Print and shaded views of the part. All mm, measured from the part's lowest x, y and z. A direction names the side the tool comes from. Coordinates: 2 decimals unless noted, no trailing zeros. Loops run counter-clockwise (first coordinate to the right, second up) from the corner with the lowest first, then second, coordinate; pieces in that order, holes last. Notation, with made-up numbers: M -4.5,16 L 5.5,16 A18 ccw 5.5,45 Z; hole C -3,30 d10. An arc over 180 degrees is marked long. Answer as a JSON object with one key per item and string values. Group by question number.
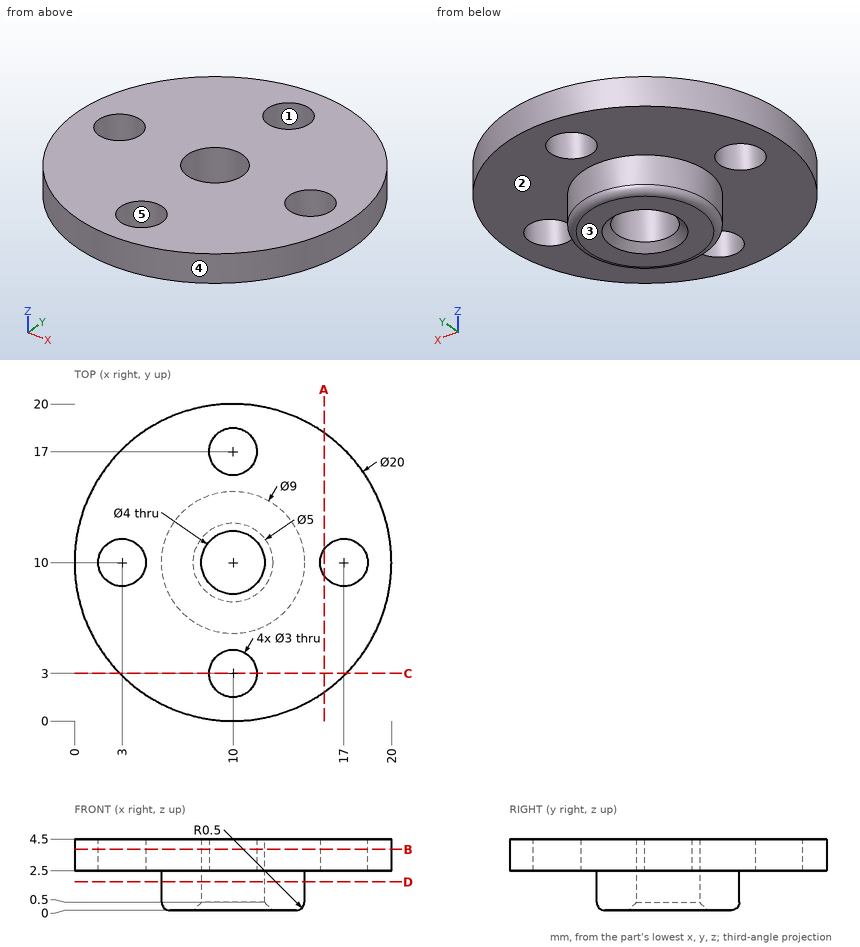
Item 1: Slice it at A-A, the plane x = 15.75. Write the cut outline in (y, z), then the cut area to 3 significant figures.
Item 2: Tool access for the marked faces 1 and 2: list every direction of +Z, -Z, +X, -X, +Y, -Y with a clear straight run to the whole face (end or side of a thin tool).
Item 3: Slice it at B-B, the plane z = 3.85. Write the cut outline in (x, y).
Item 4: Drill centre lines: L1, parallel to Z at x = 8.5, y = 15.25; L2, parallel to X at y = 2, z = 3.8; L3, parallel to Y at x = 10, z = 2.05. Where is each one in solid material? Low to high. Write a range as from..to.
Item 5: Slice it at D-D, the plane z = 1.8. Write the cut outline in (x, y).
Item 6: Pull direction Y, two halves, no side cores. Call the marked faces 3, 4 and 5: released by +Y, released by -Y, zero draft, split by the parting line, or undercut.
Item 7: Slice it at C-C, the plane y = 3. Write the cut outline in (x, z).
Item 8: Pin check, flat tips, straight feed: pin 1 (4 mm diameter, centred on x = 10, y = 17, fed in from -Z); pin 2 (1 mm diameter, centred on y = 7.5, z = 0.5, fed in from +X); pin 3 (2 mm diameter, centred on y = 6, z = 2.5, fed in from -X). Stop position of each tip, or through.
Computed:
{
 "1": {"outline": "M 1.82,2.5 L 9.17,2.5 L 9.17,4.5 L 1.82,4.5 Z; M 10.83,2.5 L 18.18,2.5 L 18.18,4.5 L 10.83,4.5 Z", "area": "29.4 mm2"},
 "2": {"face 1": "+Z, -Z", "face 2": "-Z"},
 "3": {"outline": "C 10,10 d20; hole C 3,10 d3; hole C 10,10 d4; hole C 10,3 d3; hole C 10,17 d3; hole C 17,10 d3"},
 "4": {"L1": "2.5..4.5", "L2": "4..8.88, 11.12..16", "L3": "5.5..8, 12..14.5"},
 "5": {"outline": "C 10,10 d9; hole C 10,10 d4"},
 "6": {"face 3": "zero draft", "face 4": "split by the parting line", "face 5": "undercut"},
 "7": {"outline": "M 2.86,2.5 L 8.5,2.5 L 8.5,4.5 L 2.86,4.5 Z; M 11.5,2.5 L 17.14,2.5 L 17.14,4.5 L 11.5,4.5 Z"},
 "8": {"pin 1": "z = 2.5", "pin 2": "x = 14.03", "pin 3": "x = 0.46"}
}
